Source: CAD feature listing. Evaluate the final solid. Frame: model axes, mm. Face numbers are marked on the shaded views. Round coordinates to 2 decimals unless told otherwise and drop trailing zeros. Loops run counter-clockwise (first coordinate to the right, second up) from the corner with the lowest first, then second, coordinate; pieces in that order, holes last. Notation, with made-up numbers: (-38, 9) -> (-29, 9) arc R26 ccw to (-29, 46) -> close; hole circle Ø5 at (-27, 11.25). An arc over 180 degrees is marked (long way). Write item = value, one per line.
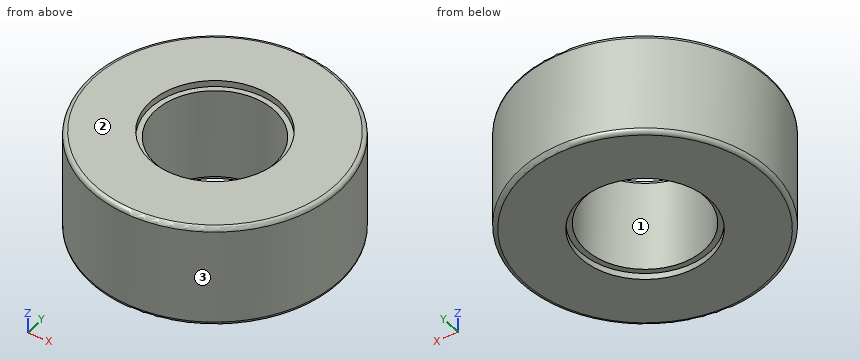
from build123d import *

# Parameters (mm, degrees)
SKETCH1_R           = 30
SKETCH1_R_2         = 14.325
BOSS_EXTRUDE1_DEPTH = 12.5
SKETCH3_R           = 15.6075
CUT_EXTRUDE1_DEPTH  = 1.524
FILLET1_R           = 1


with BuildPart() as part:
    # Sketch1 → Boss-Extrude1 (new, symmetric)
    with BuildSketch(Plane.XY):
        Circle(SKETCH1_R)
        Circle(SKETCH1_R_2, mode=Mode.SUBTRACT)
    extrude(amount=BOSS_EXTRUDE1_DEPTH, both=True)

    # Sketch3 → Cut-Extrude1 (cut)
    with BuildSketch(Plane.XY.offset(12.5)):
        Circle(SKETCH3_R)
    cut_extrude1 = extrude(amount=-CUT_EXTRUDE1_DEPTH, mode=Mode.SUBTRACT)

    # Mirror1: Cut-Extrude1 across plane
    add(cut_extrude1.mirror(Plane.XY), mode=Mode.SUBTRACT)

    # Fillet1
    fillet1_edges = [part.edges().sort_by_distance(p)[0] for p in [
        (-30, 0, -12.5),
        (-30, 0, 12.5),
    ]]
    fillet(fillet1_edges, radius=FILLET1_R)


solid = part.part
1. Mould query, pull axis Y, two halves, no side actions, for the marked faces 1, 2 and 3. Classes: released by +Y, released by -Y, zero draft, split by the parting line, or undercut.
Evaluation:
face_1 = undercut
face_2 = zero draft
face_3 = split by the parting line
2. Section query A-A (x = 0). Return the cut outline in (y, z) (1 decimal), then the cut area to 3 significant figures.
Evaluation:
outline = (-30, -11.5) arc R1 ccw to (-29, -12.5) -> (-15.6, -12.5) -> (-15.6, -11) -> (-14.3, -11) -> (-14.3, 11) -> (-15.6, 11) -> (-15.6, 12.5) -> (-29, 12.5) arc R1 ccw to (-30, 11.5) -> close; (14.3, -11) -> (15.6, -11) -> (15.6, -12.5) -> (29, -12.5) arc R1 ccw to (30, -11.5) -> (30, 11.5) arc R1 ccw to (29, 12.5) -> (15.6, 12.5) -> (15.6, 11) -> (14.3, 11) -> close
area = 775 mm²
3. Section query C-C (z = 8). Return the cut outline in (x, y) (3 decimals).
Evaluation:
outline = circle Ø60 at (0, 0); hole circle Ø28.65 at (0, 0)
4. Contact query for flat-ended pins moving along their axis: pin 1 Ø15.5 at (x, y) = (0.5, 7) entering from +Z; pin 2 Ø2 at (y, z) = (15, 1) entering from -X; pin 3 Ø18.5 at (x, y) = (0, 0) entering from -Z; pin 4 Ø4 at (x, z) = (12.5, 9) entering from -Y. Output: stop coordinate, or through.
Evaluation:
pin_1 = 10.98
pin_2 = -26.53
pin_3 = through
pin_4 = -28.1
5. Line query: probe 1 along Y at (x, z) = (0, 11.45); probe 2 along Y at (x, z) = (0, 0.5) (3 decimals); probe 3 along Z at (x, y) = (-14.5, 2.5). Output: solid intervals per line, ascending. Write a range as from..to.
Evaluation:
probe_1 = -30..-15.61, 15.61..30
probe_2 = -30..-14.325, 14.325..30
probe_3 = -10.98..10.98
